Check sheet for the modelled part. Datum: model origin and axes. Units: mm. Face numbers are marked on the shaded views. A direction names the side the tool comes from. Give positions to 0.01 mm unless a question says otherwise; leave off trailing zeros. Loops run counter-clockwise (first coordinate to the right, second up) from the corner with the lowest first, then second, coordinate; pieces in that order, holes last. Notation, with made-up numbers: M 9.5,54.5 L 40.5,54.5 A36 cw 40.5,90.5 Z; hole C -12,12 d6. An arc over 180 degrees is marked long. Use one line per item in the form item = value.
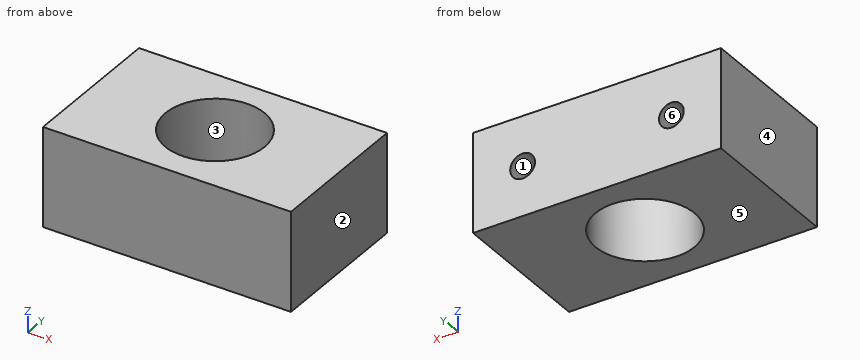
from build123d import *

# Parameters (mm, degrees)
SKETCH1_W           = 31.75
SKETCH1_H           = 19.05
BOSS_EXTRUDE1_DEPTH = 12.7
SKETCH2_R           = 6.35
CUT_EXTRUDE1_DEPTH  = 12.7
SKETCH3_R           = 1.5875
CUT_EXTRUDE2_DEPTH  = 12.7


with BuildPart() as part:
    # Sketch1 → Boss-Extrude1 (new body)
    with BuildSketch(Plane.XY):
        Rectangle(SKETCH1_W, SKETCH1_H)
    extrude(amount=BOSS_EXTRUDE1_DEPTH)

    # Sketch2 → Cut-Extrude1 (cut)
    with BuildSketch(Plane.XY.offset(12.7)):
        Circle(SKETCH2_R)
    extrude(amount=-CUT_EXTRUDE1_DEPTH, mode=Mode.SUBTRACT)

    # Sketch3 → Cut-Extrude2 (cut)
    with BuildSketch(Plane(origin=(0, 9.525, 0), x_dir=(1, 0, 0), z_dir=(0, 1, 0))):
        with Locations((-9.525, -6.35)):
            Circle(SKETCH3_R)
        with Locations((9.525, -6.35)):
            Circle(SKETCH3_R)
    extrude(amount=-CUT_EXTRUDE2_DEPTH, mode=Mode.SUBTRACT)


solid = part.part
1) Section check C-C (x = 0). Record the cut outline in (y, z) (3 decimals).
Evaluation:
outline = M -9.525,0 L -6.35,0 L -6.35,12.7 L -9.525,12.7 Z; M 6.35,0 L 9.525,0 L 9.525,12.7 L 6.35,12.7 Z
2) Scan lines: line 1 (Y direction, x = 0, z = 10.25) (3 decimals); line 2 (Z direction, x = 9.5, y = -2); line 3 (X direction, y = 0.25, z = 9.5) (3 decimals). Record each from-to range of solid material in increasing order.
Evaluation:
line_1 = -9.525 to -6.35, 6.35 to 9.525
line_2 = 0 to 4.76, 7.94 to 12.7
line_3 = -15.875 to -6.345, 6.345 to 15.875
3) Release check for a two-part mould opening along X. For the marked faces 3, 4, 5 and 6 record: pulls with the +X half, pulls with the -X half, needs draft (parallel to the pull), parting line crosses it, or undercut.
Evaluation:
face_3 = undercut
face_4 = pulls with the -X half
face_5 = needs draft
face_6 = undercut
4) Section check D-D (x = -9). Record the cut outline in (y, z) (3 decimals).
Evaluation:
outline = M -9.525,0 L 9.525,0 L 9.525,4.852 L -3.175,4.852 L -3.175,7.848 L 9.525,7.848 L 9.525,12.7 L -9.525,12.7 Z
5) Section check A-A (y = 0). State how many separate pieces and enclosed holes the cut face has, then the cut area to 3 significant figures.
Evaluation:
separate_pieces = 2
enclosed_holes = 2
area = 226 mm^2
6) Depth check by flat-ended pin: pin 1 Ø1 at (x, z) = (-10, 5.5) entering from +Y (3 decimals). Enter the tip coordinate at first touch or a pass-through.
Evaluation:
pin_1 = -3.175
7) Set-up check for the marked faces 1 and 2: record each of +Z, -Z, +X, -X, +Y, -Y from which the full face is reachable in a straight line by a thin tool's end or side.
Evaluation:
face_1 = +Y
face_2 = +Z, -Z, +X, +Y, -Y
